Here's how the part is built. I have some questions about the finished solid (model axes, mm). Face numbers are marked on the shaded views. A direction names the side the tool comes from. Coordinates: 2 decimals unless noted, no trailing zeros. Loops run counter-clockwise (first coordinate to the right, second up) from the corner with the lowest first, then second, coordinate; pieces in that order, holes last. Notation, with made-up numbers: (26, -22.75) -> (36, -22.75) arc R25 ccw to (36, -8.75) -> close; hole circle Ø6 at (-2, 87). An arc over 180 degrees is marked (long way). Answer as a JSON object with one key per item and string values. Group by question number.
Q1. I want a section at A-A on z = 50. Write out the boundary of the cut face in (x, y).
Q2. I want a section at B-B on y = 2. Write out the boundary of the cut face in (x, z).
Q3. On a 3-axis mill with a long thin cutter (end or side, diameter ignored), from which of +Z, -Z, +X, -X, +Y, -Y can I reach the whole of each face in a straight line? I mean the marked faces 1 and 2. Say none if no direction works.
Q4. Thinking about a two-plate mould opening in Z: for the marked faces 3, 4 and 5, which applies, released by +Z, released by -Z, zero draft, split by the parting line, or undercut?
Q5. I'm going to push flat-ended pins straight in: pin 1 (21.5 mm diameter, centred on x = 14, z = 49.5, fed in from +Y); pin 2 (4 mm diameter, centred on x = 16, z = -71, fed in from -Y). Where does each tip first touch, or does it pass through?
Q6. I need wall thicknesses on line 1 (X direction, y = -12, z = 50); line 2 (Y direction, x = -32, z = 45.5); line 3 (X direction, y = -2.7, z = -50). Which ranges of each line are inside material? Lowest first, please.
Q7. I want a section at C-C on x = 0. Count the separate pieces of the cut face and the enclosed holes in it, then the cut area to 3 significant figures.
Q8. I want a section at D-D on z = -51. Write out the boundary of the cut face in (x, y).
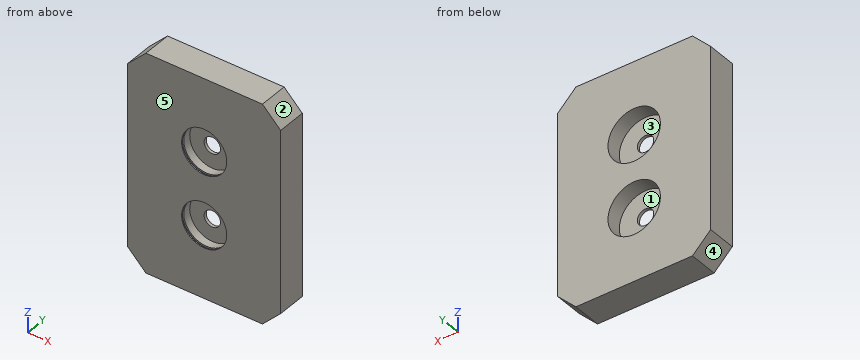
```python
from build123d import *

# Parameters (mm, degrees)
F1_DEPTH = 20
F2_W     = 3.0358287096
F2_H     = 31
F2_W_2   = 4
F2_H_2   = 11.25


# Not quite as in the source:
# - a pattern or mirror of a feature is missing from the dataset's text; its kind, count and spacing are read off the source's solid


with BuildPart() as f1:
    # F0 (on Front) → F1 (new body, symmetric)
    with BuildSketch(Plane.XZ):
        Polygon((80, 150), (-80, 150), (-105, 125), (-105, -125), (-80, -150), (80, -150), (105, -125), (105, 125), align=None)
    extrude(amount=F1_DEPTH, both=True)

    # F2 (on Right) → F3 (revolve, cut)
    with BuildSketch(Plane.YZ):
        with Locations((-20.0179143548, 65.5)):
            Rectangle(F2_W, F2_H)
        Polygon((-18.5, 81), (-18.5, 50), (-16, 50), (-16, 81), (-16, 83), (-18.5, 83), align=None)
        Polygon((-16, 81), (-16, 50), (-5, 50), (-5, 61.25), (-5, 81), align=None)
        with Locations((-3, 55.625)):
            Rectangle(F2_W_2, F2_H_2)
        Polygon((-1, 61.25), (-1, 50), (34.8119065166, 50), (34.8119065166, 86), (-1, 86), align=None)
    f3 = revolve(axis=Axis((0, 5.6746993214, 50), (0, 1, 0)), mode=Mode.SUBTRACT)

    # F3_copies: F3 across plane
    add(f3.mirror(Plane(origin=(0, 0, 0), x_dir=(-1, 0, 0), z_dir=(0, 0, -1))), mode=Mode.SUBTRACT)


solid = f1.part
```
Result set:
{
 "1": {"outline": "(-105, -20) -> (-31, -20) -> (-31, -18.5) -> (-33, -18.5) -> (-33, -16) -> (-31, -16) -> (-31, -5) -> (-11.25, -5) -> (-11.25, -1) -> (-36, -1) -> (-36, 20) -> (-105, 20) -> close; (11.25, -5) -> (31, -5) -> (31, -16) -> (33, -16) -> (33, -18.5) -> (31, -18.5) -> (31, -20) -> (105, -20) -> (105, 20) -> (36, 20) -> (36, -1) -> (11.25, -1) -> close"},
 "2": {"outline": "(-105, -125) -> (-80, -150) -> (80, -150) -> (105, -125) -> (105, 125) -> (80, 150) -> (-80, 150) -> (-105, 125) -> close; hole circle Ø72 at (0, -50); hole circle Ø72 at (0, 50)"},
 "3": {"face 1": "+Y", "face 2": "+Z, +X, +Y, -Y"},
 "4": {"face 3": "undercut", "face 4": "released by -Z", "face 5": "zero draft"},
 "5": {"pin 1": "stops at y = -1", "pin 2": "stops at y = -5"},
 "6": {"line 1": "x = -105 to -31, 31 to 105", "line 2": "y = -20 to -18.5, -16 to -1", "line 3": "x = -105 to -11.25, 11.25 to 105"},
 "7": {"separate pieces": "3", "enclosed holes": "0", "area": "6,920 mm²"},
 "8": {"outline": "(-105, -20) -> (-30.98, -20) -> (-30.98, -18.5) -> (-32.98, -18.5) -> (-32.98, -16) -> (-30.98, -16) -> (-30.98, -5) -> (-11.21, -5) -> (-11.21, -1) -> (-35.99, -1) -> (-35.99, 20) -> (-105, 20) -> close; (11.21, -5) -> (30.98, -5) -> (30.98, -16) -> (32.98, -16) -> (32.98, -18.5) -> (30.98, -18.5) -> (30.98, -20) -> (105, -20) -> (105, 20) -> (35.99, 20) -> (35.99, -1) -> (11.21, -1) -> close"}
}
